from build123d import *

# Parameters (mm, degrees)
F1_DEPTH = 6
F2_R     = 1.5
F4_DEPTH = 6
F5_DEPTH = 4
F6_R     = 1.45
F7_DEPTH = 8


with BuildPart() as f1:
    # F0 (on Front) → F1 (new body)
    with BuildSketch(Plane.XZ):
        Polygon((0, 0), (0, -12.2), (-10.1, -12.2), (-10.1, -10.7), (-14, -14.7), (2.5, -14.7), (2.5, 0), (6, 0), (6, 2.5), (-14, 2.5), (-10.1, -1.5), (-10.1, 0), align=None)
    extrude(amount=F1_DEPTH)

    # F2
    f2_edges = [f1.edges().sort_by_distance(p)[0] for p in [
        (-14, -3, -14.7),
        (-14, -3, 2.5),
    ]]
    fillet(f2_edges, radius=F2_R)

    # F3 (on face) → F4 (join)
    with BuildSketch(Plane(origin=(0, 0, 0), x_dir=(1, 0, 0), z_dir=(0, 0, -1))):
        with BuildLine():
            Line((2.5, 0), (5.1113989637, 1.4766839378))
            ThreePointArc((5.1113989637, 1.4766839378), (5.7616130766, 2.1182257053), (6, 3))
            ThreePointArc((6, 3), (5.7616130766, 3.8817742947), (5.1113989637, 4.5233160622))
            Line((5.1113989637, 4.5233160622), (2.5, 6))
            Line((2.5, 6), (2.5, 0))
        make_face()
    extrude(amount=F4_DEPTH)

    # F5 (cut): faces of the model
    f5_faces = [f1.faces().sort_by_distance(p)[0] for p in [
        (4.8789891279, -0.7262583823, 0),
        (4.8789891279, -5.2737416177, 0),
    ]]
    extrude(f5_faces, amount=-F5_DEPTH, mode=Mode.SUBTRACT)

    # F6 (on face) → F7 (cut)
    with BuildSketch(Plane.XY.offset(2.5)):
        with Locations((2.8, -3)):
            Circle(F6_R)
    extrude(amount=-F7_DEPTH, mode=Mode.SUBTRACT)


solid = f1.part
Part model, mm, in its own coordinate system. A direction names the side the tool comes from. Coordinates: 2 decimals unless noted, no trailing zeros. Loops run counter-clockwise (first coordinate to the right, second up) from the corner with the lowest first, then second, coordinate; pieces in that order, holes last. Notation, with made-up numbers: (2.5, 59) - (49.5, 59) arc R23 ccw to (49.5, 97) - close; hole circle Ø9 at (-29, 12). An arc over 180 degrees is marked (long way). Write each question's results on one line, items separated by ' | '. Start each with the question number.
Q1. Which spindle directions (+Z, -Z, +X, -X, +Y, -Y) get a long thin tool onto all of the face, cutting with end or side? Do faces 1 (the flat face through (-10.1, -3, -1)), 2 (the cylindrical face through (1.73, -2.02, -1.44)), 3 (the flat face through (-4, -3, 2.5)), 4 (the flat face through (-10.8, -2.96, -11.42)), 5 (the cylindrical face through (6, -3, -2)). Say none if no direction does.
Q2. Probe line 1 along X through (y, z) = (-3.3, -0.75); line 2 along Z through (x, y) = (-5.5, -4.5); line 3 along X through (y, z) = (-4.15, -11.75). List the from-to ranges inside material, lowest first.
Q3. Slice it at C-C on z = -8.25. Give the cut face in (x, y), and give its area (3 significant figures).
Q4. Slice it at B-B on x = -6.5. Give the cut face in (y, z), and give its area (3 significant figures).
Q5. Slice it at A-A on z = -4. Give the cut face in (x, y).
Q6. Drop flat-ended pins along their axis: pin 1 Ø0.8 at (y, z) = (-2, -11.5) entering from +X; pin 2 Ø3 at (y, z) = (-4.5, -12.5) entering from -X; pin 3 Ø1.5 at (x, y) = (3, -3.5) entering from +Z; pin 4 Ø1.5 at (y, z) = (-2.5, -9.5) entering from -X. Give the stop position or say it passes through.
Q7. Two-plate mould, pull along Y, no slides. Class faces 6 (the flat face through (3, -3, -5.5)), 7 (the flat face through (1, 0, -5)), 8 (the flat face through (3.824, -5.251, -1.69)), 9 (the flat face through (4, -3, -6)): +Y half, -Y half, draft (parallel to the pull), parting line (faces both ways), or undercut.
Q8. Slice it at D-D on x = 2.8. Give the cut face in (y, z).
Answer:
1) face 1: +Y, -Y | face 2: +Z | face 3: +Z, +X, -X, +Y, -Y | face 4: -X, +Y, -Y | face 5: +Z, -Z, +X
2) line 1: x = -10.83 to -10.1, 0 to 1.38, 4.22 to 5.97 | line 2: z = -14.7 to -12.2, 0 to 2.5 | line 3: x = -11.12 to -10.1, 0 to 2.5
3) outline: (0, -6) - (2.5, -6) - (2.5, 0) - (0, 0) - close | area: 15.0 mm2
4) outline: (-6, -14.7) - (0, -14.7) - (0, -12.2) - (-6, -12.2) - close; (-6, 0) - (0, 0) - (0, 2.5) - (-6, 2.5) - close | area: 30.0 mm2
5) outline: (0, -6) - (2.5, -6) - (5.11, -4.52) arc R1.75 ccw to (5.11, -1.48) - (2.5, 0) - (0, 0) - close; hole circle Ø2.9 at (2.8, -3)
6) pin 1: stops at x = 2.5 | pin 2: stops at x = -11.94 | pin 3: stops at z = -5.5 | pin 4: stops at x = 0
7) face 6: undercut | face 7: +Y half | face 8: -Y half | face 9: draft
8) outline: (-5.83, -6) - (-0.17, -6) - (-0.17, 2.5) - (-1.55, 2.5) - (-1.55, -5.5) - (-4.45, -5.5) - (-4.45, 2.5) - (-5.83, 2.5) - close
